```python
from build123d import *

# Parameters (mm, degrees)
SKETCH_1_W                         = 55.6
SKETCH_1_H                         = 20
SM_BASE_FLANGE_1_DEPTH             = 2
SM_EDGE_FLANGE_1_STRIP_W           = 9.4732
SM_EDGE_FLANGE_1_STRIP_H           = 2
SM_EDGE_FLANGE_1_STRIP_CUT_DEPTH   = 20
SM_EDGE_FLANGE_1_STRIP_2_W         = 9.4732
SM_EDGE_FLANGE_1_STRIP_2_H         = 2
SM_EDGE_FLANGE_1_STRIP_CUT_2_DEPTH = 20
SM_EDGE_FLANGE_1_DEPTH             = 20
SM_EDGE_FLANGE_1_BEND_DEPTH        = 20
SKETCH_12_R                        = 1.5
CUT_EXTRUDE_1_DEPTH                = 67.45569953
SKETCH_13_R                        = 3
SKETCH_13_R_2                      = 1.5
CUT_EXTRUDE_2_DEPTH                = 48.348072822


# Sheet-metal steps are written as plain solids
with BuildPart() as part:
    # Sketch 1 → 基体-法兰1 (new body)
    with BuildSketch(Plane(origin=(0, 0, 0), x_dir=(1, 0, 0), z_dir=(0, 1, 0))):
        Rectangle(SKETCH_1_W, SKETCH_1_H)
    extrude(amount=-SM_BASE_FLANGE_1_DEPTH)

    # 边线-法兰1 strip (across the edge) → 边线-法兰1 strip cut (cut)
    with BuildSketch(Plane(origin=(-27.8, 0, -10), x_dir=(1, 0, 0), z_dir=(0, 0, 1))):
        with Locations((-2, -1)):
            Rectangle(SM_EDGE_FLANGE_1_STRIP_W, SM_EDGE_FLANGE_1_STRIP_H)
    extrude(amount=SM_EDGE_FLANGE_1_STRIP_CUT_DEPTH, mode=Mode.SUBTRACT)

    # 边线-法兰1 strip 2 (across the edge) → 边线-法兰1 strip cut 2 (cut)
    with BuildSketch(Plane(origin=(27.8, 0, 10), x_dir=(-1, 0, 0), z_dir=(0, 0, -1))):
        with Locations((-2, -1)):
            Rectangle(SM_EDGE_FLANGE_1_STRIP_2_W, SM_EDGE_FLANGE_1_STRIP_2_H)
    extrude(amount=SM_EDGE_FLANGE_1_STRIP_CUT_2_DEPTH, mode=Mode.SUBTRACT)

    # 边线-法兰1 section (across the edge) → 边线-法兰1 (add)
    with BuildSketch(Plane(origin=(-27.8, 0, -10), x_dir=(1, 0, 0), z_dir=(0, 0, 1))):
        with BuildLine():
            Line((0, 0.7366), (0, 35))
            Line((0, 35), (2, 35))
            Line((2, 35), (2, 0.7366))
            ThreePointArc((2, 0.7366), (2.215745145, 0.215745145), (2.7366, 0))
            Line((2.7366, 0), (2.7366, -2))
            ThreePointArc((2.7366, -2), (0.801531583, -1.198468417), (0, 0.7366))
        make_face()
    extrude(amount=SM_EDGE_FLANGE_1_DEPTH)

    # 边线-法兰1 section 2 (across the edge) → 边线-法兰1 bend (add)
    with BuildSketch(Plane(origin=(27.8, 0, 10), x_dir=(-1, 0, 0), z_dir=(0, 0, -1))):
        with BuildLine():
            Line((0, 0.7366), (0, 35))
            Line((0, 35), (2, 35))
            Line((2, 35), (2, 0.7366))
            ThreePointArc((2, 0.7366), (2.215745145, 0.215745145), (2.7366, 0))
            Line((2.7366, 0), (2.7366, -2))
            ThreePointArc((2.7366, -2), (0.801531583, -1.198468417), (0, 0.7366))
        make_face()
    extrude(amount=SM_EDGE_FLANGE_1_BEND_DEPTH)

    # 草图12 → 切除-拉伸1 (cut, through all)
    with BuildSketch(Plane(origin=(27.8, 0, 0), x_dir=(0, 0, -1), z_dir=(1, 0, 0))):
        with BuildLine():
            Line((-10, 35), (-10, 25))
            ThreePointArc((-10, 25), (-7.071067812, 32.071067812), (0, 35))
            Line((0, 35), (-10, 35))
        make_face()
        with BuildLine():
            ThreePointArc((0, 35), (7.071067812, 32.071067812), (10, 25))
            Line((10, 25), (10, 35))
            Line((10, 35), (0, 35))
        make_face()
        with BuildLine():
            ThreePointArc((0, 29), (-4, 25), (0, 21))
            Line((0, 21), (0, 29))
        make_face()
        with BuildLine():
            Line((0, 29), (0, 21))
            ThreePointArc((0, 21), (2.828427125, 22.171572875), (4, 25))
            ThreePointArc((4, 25), (2.828427125, 27.828427125), (0, 29))
        make_face()
        with Locations(Location((-7, 25, 0), (0, 0, 90))):
            Circle(SKETCH_12_R)
        with Locations(Location((-4.949747468, 20.050252532, 0), (0, 0, 90))):
            Circle(SKETCH_12_R)
        with Locations(Location((0, 18, 0), (0, 0, 90))):
            Circle(SKETCH_12_R)
        with Locations(Location((4.949747468, 20.050252532, 0), (0, 0, 90))):
            Circle(SKETCH_12_R)
        with Locations(Location((7, 25, 0), (0, 0, 90))):
            Circle(SKETCH_12_R)
        with Locations(Location((0, 32, 0), (0, 0, 90))):
            Circle(SKETCH_12_R)
    extrude(amount=-CUT_EXTRUDE_1_DEPTH, mode=Mode.SUBTRACT)

    # 草图13 → 切除-拉伸2 (cut, through all)
    with BuildSketch(Plane.XZ.offset(2)):
        with Locations(Location((0, 0, 0), (0, 0, 270))):
            Circle(SKETCH_13_R)
        with Locations(Location((-15, 5, 0), (0, 0, 270))):
            Circle(SKETCH_13_R_2)
        with Locations(Location((-5, 5, 0), (0, 0, 270))):
            Circle(SKETCH_13_R_2)
        with Locations(Location((5, 5, 0), (0, 0, 270))):
            Circle(SKETCH_13_R_2)
        with Locations(Location((15, 5, 0), (0, 0, 270))):
            Circle(SKETCH_13_R_2)
        with Locations(Location((-5, -5, 0), (0, 0, 270))):
            Circle(SKETCH_13_R_2)
        with Locations(Location((5, -5, 0), (0, 0, 270))):
            Circle(SKETCH_13_R_2)
        with Locations(Location((15, -5, 0), (0, 0, 270))):
            Circle(SKETCH_13_R_2)
        with Locations(Location((-15, -5, 0), (0, 0, 270))):
            Circle(SKETCH_13_R_2)
    extrude(amount=-CUT_EXTRUDE_2_DEPTH, mode=Mode.SUBTRACT)


solid = part.part
```
For this review, take the finished solid that the model builds, in its own axes (mm). A direction names the side the tool comes from. Round coordinates to 2 decimals unless told otherwise and drop trailing zeros. Write each loop counter-clockwise with the first axis right and the second up, starting at its lowest first coordinate (ties: lowest second). Pieces come first, ordered by that corner, then holes. Notation, with made-up numbers: (19.5, -16) -> (24.5, -16) arc R34 cw to (24.5, 19) -> close; hole circle Ø10 at (64.5, 66). An arc over 180 degrees is marked (long way). Use one line per item in the form item = value.
1) Take a section at D-D, the plane y = 32. Write out the cut boundary in (x, z).
Found:
outline = (-27.8, -7.14) -> (-25.8, -7.14) -> (-25.8, -1.5) -> (-27.8, -1.5) -> close; (-27.8, 1.5) -> (-25.8, 1.5) -> (-25.8, 7.14) -> (-27.8, 7.14) -> close; (25.8, -7.14) -> (27.8, -7.14) -> (27.8, -1.5) -> (25.8, -1.5) -> close; (25.8, 1.5) -> (27.8, 1.5) -> (27.8, 7.14) -> (25.8, 7.14) -> close
2) To check wall thickness, follow L1, parallel to X at y = 4, z = 7.5; L2, parallel to X at y = -0.85, z = 5; L3, parallel to Y at x = 22, z = -1.75. State the ranges of each line that lie inside material, in increasing order. Write a range as from..to.
Found:
L1 = -27.8..-25.8, 25.8..27.8
L2 = -27.29..-16.5, -13.5..-6.5, -3.5..3.5, 6.5..13.5, 16.5..27.29
L3 = -2..0
3) Clearance check with flat-ended pins moving along their axes: pin 1 (4 mm diameter, centred on x = -5, z = -5, fed in from +Y); pin 2 (1 mm diameter, centred on y = 24.5, z = -7, fed in from -X). State where each tip first meets the part, or that it passes through.
Found:
pin_1 = 0
pin_2 = through
4) Take a section at A-A, the plane x = 0. Write out the cut boundary in (y, z), and give its area (3 significant figures).
Found:
outline = (-2, -10) -> (0, -10) -> (0, -3) -> (-2, -3) -> close; (-2, 3) -> (0, 3) -> (0, 10) -> (-2, 10) -> close
area = 28.0 mm2
5) Mouldability with a two-part tool opening along X and no side actions: class faces 1 (the cylindrical face through (-14.93, -1.01, 6.5)), 2 (the cylindrical face through (26.81, 16.5, 0.07)), 3 (the cylindrical face through (26.977, -1.22, 0.14)) as +X half, -X half, draft (parallel to the pull), parting line (faces both ways), or undercut.
Found:
face_1 = undercut
face_2 = draft
face_3 = +X half
6) Tool access review of faces 4 (the cylindrical face through (4.425, -1.014, -6.386)), 5 (the flat face through (-25.8, 14, 0)): name each direction out of +Z, -Z, +X, -X, +Y, -Y from which nothing blocks a thin tool from reaching the whole face with its end or side.
Found:
face_4 = +Y, -Y
face_5 = +Z, -Z, +Y
7) Take a section at C-C, the plane x = 15. Write out the cut boundary in (y, z), and give its area (3 significant figures).
Found:
outline = (-2, -10) -> (0, -10) -> (0, -6.5) -> (-2, -6.5) -> close; (-2, -3.5) -> (0, -3.5) -> (0, 3.5) -> (-2, 3.5) -> close; (-2, 6.5) -> (0, 6.5) -> (0, 10) -> (-2, 10) -> close
area = 28.0 mm2
8) Take a section at B-B, the plane y = 5. Write out the cut boundary in (x, z), and give its area (3 significant figures).
Found:
outline = (-27.8, -10) -> (-25.8, -10) -> (-25.8, 10) -> (-27.8, 10) -> close; (25.8, -10) -> (27.8, -10) -> (27.8, 10) -> (25.8, 10) -> close
area = 80.0 mm2
